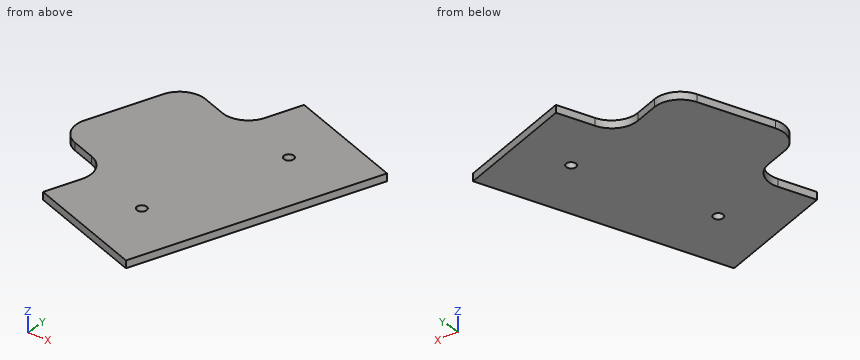
from build123d import *

# Parameters (mm, degrees)
EXTRUDE_1_DEPTH     = 3
CUT_EXTRUDE_1_REACH = 877.393
SKETCH_2_R          = 1.95
EXTRUDE_2_DEPTH     = 3
FILLET_1_R          = 10


with BuildPart() as part:
    # 草图1 → 凸台-拉伸1 (new body)
    with BuildSketch(Plane.XY):
        Polygon((366.808331571, 667.065590198), (401.010345904, 761.034852277), (354.025714865, 778.135859443), (319.823700532, 684.166597365), align=None)
    extrude(amount=EXTRUDE_1_DEPTH)

    # 草图2 → 切除-拉伸1 (cut, up to next)
    with BuildSketch(Plane.XY.offset(3), mode=Mode.PRIVATE) as cut_extrude_1_sk1:
        with Locations((351.338243096, 695.576064033)):
            Circle(SKETCH_2_R)
    cut_extrude_1_tool1 = extrude(cut_extrude_1_sk1.sketch, amount=-CUT_EXTRUDE_1_REACH, mode=Mode.PRIVATE) & part.part
    # 草图2 → 切除-拉伸1 (cut, up to next)
    with BuildSketch(Plane.XY.offset(3), mode=Mode.PRIVATE) as cut_extrude_1_sk2:
        with Locations((369.862047426, 749.482173827)):
            Circle(SKETCH_2_R)
    cut_extrude_1_tool2 = extrude(cut_extrude_1_sk2.sketch, amount=-CUT_EXTRUDE_1_REACH, mode=Mode.PRIVATE) & part.part
    add(cut_extrude_1_tool1.solids().sort_by_distance((351.338243, 695.576064, 3))[0], mode=Mode.SUBTRACT)
    add(cut_extrude_1_tool2.solids().sort_by_distance((369.862047, 749.482174, 3))[0], mode=Mode.SUBTRACT)

    # 草图3 → 凸台-拉伸2 (add)
    with BuildSketch(Plane.XY.offset(3)):
        Polygon((345.475211281, 754.643543924), (317.284432658, 764.904148223), (300.183425492, 717.919517184), (328.374204115, 707.658912884), align=None)
    extrude(amount=-EXTRUDE_2_DEPTH)

    # 圆角1
    fillet_1_edges = [part.edges().sort_by_distance(p)[0] for p in [
        (345.475211281, 754.643543924, 1.5),
        (328.374204115, 707.658912884, 1.5),
        (300.183425492, 717.919517184, 1.5),
        (317.284432658, 764.904148223, 1.5),
    ]]
    fillet(fillet_1_edges, radius=FILLET_1_R)


solid = part.part
Build history of the part. All positions in model axes, mm. Coordinates: 2 decimals unless noted, no trailing zeros. Write each loop counter-clockwise with the first axis right and the second up, starting at its lowest first coordinate (ties: lowest second). Pieces come first, ordered by that corner, then holes.
(1) Cut at A-A on z = 2.55. List the corners of the cut face in (x, y), and give its area (3 significant figures).
(2) Drill centre lines: line 1 (X direction, y = 694, z = 1.35); line 2 (Y direction, x = 360, z = 2.5); line 3 (X direction, y = 704, z = 1.15). Where is each one in solid material? Low to high.
(3) Cut at C-C on x = 384.5. List the corners of the cut face in (y, z).
(4) Cut at B-B on y = 704. List the corners of the cut face in (x, z).
Working result:
1. outline: (303.6, 727.32) arc R10 ccw to (309.58, 714.5) - (318.98, 711.08) arc R10 cw to (324.95, 698.26) - (319.82, 684.17) - (366.81, 667.07) - (401.01, 761.03) - (354.03, 778.14) - (348.9, 764.04) arc R10 cw to (336.08, 758.06) - (326.68, 761.48) arc R10 ccw to (313.86, 755.51) - close; hole circle Ø3.9 at (351.34, 695.58); hole circle Ø3.9 at (369.86, 749.48)
1. area: 6,480 mm2
2. line 1: x = 323.4 to 350.19, 352.49 to 376.61
2. line 2: y = 669.54 to 775.96
2. line 3: x = 325.28 to 380.25
3. outline: (715.67, 0) - (767.04, 0) - (767.04, 3) - (715.67, 3) - close
4. outline: (325.28, 0) - (380.25, 0) - (380.25, 3) - (325.28, 3) - close
